from build123d import *

# Parameters (mm, degrees)
SKETCH1_W                    = 25.4
SKETCH1_H                    = 25.4
SKETCH1_W_2                  = 19.05
SKETCH1_H_2                  = 19.05
BOSS_EXTRUDE1_DEPTH          = 304.8
CUT_EXTRUDE3_REACH           = 308.12
SKETCH4_W                    = 19.05
SKETCH4_H                    = 28.575
F_3_8_CLEARANCE_HOLE1_D      = 10.0838
F_1_8_0_125_DIAMETER_HOLE1_D = 3.175
F_10_CLEARANCE_HOLE1_D       = 5.1054
FILLET1_R                    = 4.7625
CUT_EXTRUDE4_DEPTH           = 307.120058147


with BuildPart() as part:
    # Sketch1 → Boss-Extrude1 (new body)
    with BuildSketch(Plane(origin=(0, 0, 0), x_dir=(1, 0, 0), z_dir=(0, 1, 0))):
        Rectangle(SKETCH1_W, SKETCH1_H)
        Rectangle(SKETCH1_W_2, SKETCH1_H_2, mode=Mode.SUBTRACT)
    extrude(amount=BOSS_EXTRUDE1_DEPTH)

    # Sketch4 → Cut-Extrude3 (cut, up to next)
    with BuildSketch(Plane.ZY.offset(12.7), mode=Mode.PRIVATE) as cut_extrude3_sk1:
        with Locations((0, 266.7)):
            Rectangle(SKETCH4_W, SKETCH4_H)
    cut_extrude3_tool1 = extrude(cut_extrude3_sk1.sketch, amount=-CUT_EXTRUDE3_REACH, mode=Mode.PRIVATE) & part.part
    # Sketch4 → Cut-Extrude3 (cut, up to next)
    with BuildSketch(Plane.ZY.offset(12.7), mode=Mode.PRIVATE) as cut_extrude3_sk2:
        with Locations((0, 38.1)):
            Rectangle(SKETCH4_W, SKETCH4_H)
    cut_extrude3_tool2 = extrude(cut_extrude3_sk2.sketch, amount=-CUT_EXTRUDE3_REACH, mode=Mode.PRIVATE) & part.part
    add(cut_extrude3_tool1.solids().sort_by_distance((-12.7, 266.7, 0))[0], mode=Mode.SUBTRACT)
    add(cut_extrude3_tool2.solids().sort_by_distance((-12.7, 38.1, 0))[0], mode=Mode.SUBTRACT)

    # 3/8 Clearance Hole1 (through all)
    with Locations(Plane.XY.offset(12.7)):
        with Locations((-6.35, 266.7), (-6.35, 38.1)):
            Hole(F_3_8_CLEARANCE_HOLE1_D / 2)

    # 1/8 (0.125) Diameter Hole1 (through all)
    with Locations(Plane.ZY.offset(12.7)):
        with Locations((6.35, 6.35), (6.35, 285.75), (-6.35, 298.45), (-6.35, 285.75), (6.35, 298.45), (6.35, 19.05), (-6.35, 19.05), (-6.35, 6.35)):
            Hole(F_1_8_0_125_DIAMETER_HOLE1_D / 2)

    # #10 Clearance Hole1 (through all)
    with Locations(Plane.XY.offset(12.7)):
        with Locations((0, 63.5), (0, 88.9), (0, 241.3), (0, 215.9)):
            Hole(F_10_CLEARANCE_HOLE1_D / 2)

    # Fillet1
    fillet1_edges = [part.edges().sort_by_distance(p)[0] for p in [
        (-11.1125, 280.9875, -9.525),
        (-11.1125, 252.4125, -9.525),
        (-11.1125, 252.4125, 9.525),
        (-11.1125, 280.9875, 9.525),
        (-11.1125, 52.3875, 9.525),
        (-11.1125, 52.3875, -9.525),
        (-11.1125, 23.8125, -9.525),
        (-11.1125, 23.8125, 9.525),
    ]]
    fillet(fillet1_edges, radius=FILLET1_R)

    # Sketch11 → Cut-Extrude4 (cut, through all)
    with BuildSketch(Plane.XY.offset(12.7)):
        with BuildLine():
            Line((-6.35, 261.6581), (-12.7, 261.6581))
            ThreePointArc((-12.7, 261.6581), (-17.7419, 266.7), (-12.7, 271.7419))
            Line((-12.7, 271.7419), (-6.35, 271.7419))
            ThreePointArc((-6.35, 271.7419), (-1.3081, 266.7), (-6.35, 261.6581))
        make_face()
        with BuildLine():
            Line((-6.35, 33.0581), (-12.7, 33.0581))
            ThreePointArc((-12.7, 33.0581), (-17.7419, 38.1), (-12.7, 43.1419))
            Line((-12.7, 43.1419), (-6.35, 43.1419))
            ThreePointArc((-6.35, 43.1419), (-1.3081, 38.1), (-6.35, 33.0581))
        make_face()
    extrude(amount=-CUT_EXTRUDE4_DEPTH, mode=Mode.SUBTRACT)


solid = part.part
The listing builds one solid part. Answer for the finished solid, in the listing's coordinates (mm). A direction names the side the tool comes from. Give positions to 0.01 mm unless a question says otherwise; leave off trailing zeros. Write each loop counter-clockwise with the first axis right and the second up, starting at its lowest first coordinate (ties: lowest second). Pieces come first, ordered by that corner, then holes.
1) For a pull along X with two mould halves and no side action, classify faces 4 (the face through (-1.178, 86.635, -11.135)), 5 (the face through (-11.09, 253.77, -8.09)), 6 (the face through (12.7, 150, 0)) as pulls with the +X half, pulls with the -X half, needs draft (parallel to the pull), parting line crosses it, or undercut.
2) Section B-B (y = 241.3) is taken. Write down the section's boundary in (x, z) (3 decimals).
3) A tool of negligible diameter and unlimited length cuts with its end or side. For faces 1 (the face through (-1.31, 266.81, 11.09)), 2 (the face through (-9.525, 11, 0)), 3 (the face through (-11.09, 25.245, -8.167)), from which of +Z, -Z, +X, -X, +Y, -Y can it reach the whole face along a straight path? Write none if from no direction.
4) Given P1, Ø3, axis at x = 0, y = 63.5, coming from the -Z side, flat-ended and moving along its own axis, determine where the tip first touches the part or whether it passes through.
5) Section C-C (y = 83.5) is taken. Write down the section's boundary in (x, z) (3 decimals), and give its area (3 significant figures).
6) Find the intervals of material crossed by L1, parallel to Z at x = -11.95, y = 298.45; L2, parallel to Y at x = 12, z = -6.35; L3, parallel to Y at x = 0, z = -11.7, in increasing order.
7) Section A-A (z = -0.5) is taken. Write down the section's boundary in (x, y) (1 decimal), and give its area (3 significant figures).
Response:
1. face 4: undercut
1. face 5: needs draft
1. face 6: pulls with the +X half
2. outline: (-12.7, -12.7) - (-2.553, -12.7) - (-2.553, -9.525) - (-9.525, -9.525) - (-9.525, 9.525) - (-2.553, 9.525) - (-2.553, 12.7) - (-12.7, 12.7) - close; (2.553, -12.7) - (12.7, -12.7) - (12.7, 12.7) - (2.553, 12.7) - (2.553, 9.525) - (9.525, 9.525) - (9.525, -9.525) - (2.553, -9.525) - close
3. face 1: +Z, -Z, -X
3. face 2: +Y, -Y
3. face 3: -X
4. P1: passes through
5. outline: (-12.7, -12.7) - (12.7, -12.7) - (12.7, 12.7) - (-12.7, 12.7) - close; hole (-9.525, -9.525) - (9.525, -9.525) - (9.525, 9.525) - (-9.525, 9.525) - close
5. area: 282 mm2
6. L1: z = -12.7 to -7.94, -4.76 to 4.76, 7.94 to 12.7
6. L2: y = 0 to 4.76, 7.94 to 17.46, 20.64 to 284.16, 287.34 to 296.86, 300.04 to 304.8
6. L3: y = 0 to 60.95, 66.05 to 86.35, 91.45 to 213.35, 218.45 to 238.75, 243.85 to 304.8
7. outline: (-12.7, 0) - (-9.5, 0) - (-9.5, 23.8) - (-12.7, 23.8) - close; (-12.7, 52.4) - (-9.5, 52.4) - (-9.5, 252.4) - (-12.7, 252.4) - close; (-12.7, 281) - (-9.5, 281) - (-9.5, 304.8) - (-12.7, 304.8) - close; (9.5, 0) - (12.7, 0) - (12.7, 304.8) - (9.5, 304.8) - close
7. area: 1,750 mm2
